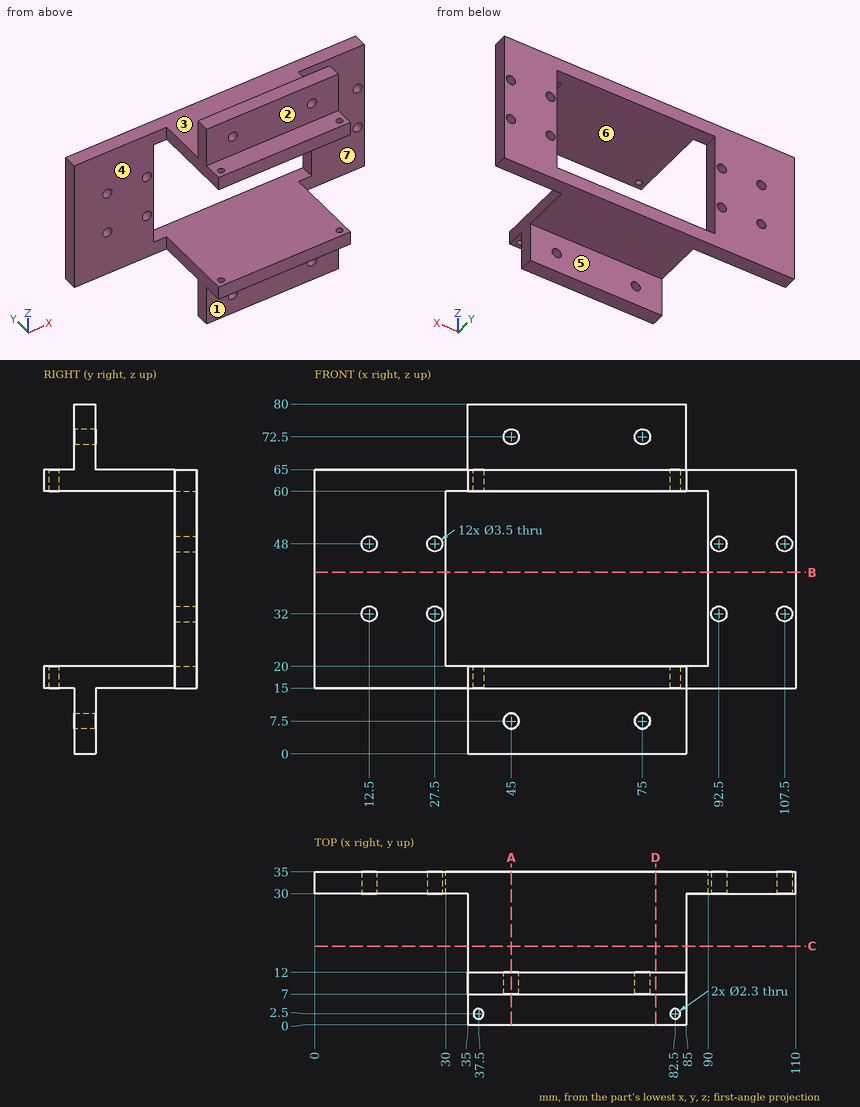
Could you check a few things on this drawing? It's one solid part, dimensions in mm from its lowest x, y, z. A direction names the side the tool comes from. Coordinates: 2 decimals unless noted, no trailing zeros. Order: outer loops, then holes, each group sorted by start corner. A loop starts at its lowest first (then second) coordinate and runs counter-clockwise, first axis right, second up. Notation, with made-up numbers: (30, -27) - (72, -27) arc R12 cw to (72, -9) - close; hole circle Ø11 at (12.25, 60). An arc over 180 degrees is marked (long way). One line per question, with ' | ' between items. Start each with the question number.
1. I'm going to push flat-ended pins straight in: pin 1 Ø5.5 at (x, y) = (51.5, 2) entering from -Z; pin 2 Ø3 at (x, z) = (12.5, 48) entering from +Y; pin 3 Ø10.5 at (x, z) = (9.5, 30) entering from -Y; pin 4 Ø12 at (x, z) = (49, 8) entering from -Y. Where does each tip first touch, or does it pass through?
2. If we section it at D-D (x = 78): Write out the boundary of the cut face in (y, z).
3. If we section it at B-B (z = 41.5): Write out the boundary of the cut face in (x, y), and give its area (3 significant figures).
4. If we mould it in two halves opening along X, with no side actions, what happens to the marked faces 6 and 7? For each: released by +X, released by -X, zero draft, split by the parting line, or undercut.
5. Which directions (+Z, -Z, +X, -X, +Y, -Y) give clear straight access to the entire face, cutting with the end or side of a thin tool? Please do the marked faces 1, 2, 3, 4 and 5.
6. Please list where these lines run through material, in increasing order: line 1 along X through (y, z) = (10.75, 72.5); line 2 along Z through (x, y) = (75, 9); line 3 along X through (y, z) = (31.45, 48). Write a range as [from, to].
7. If we section it at A-A (x = 45): Write out the boundary of the cut face in (y, z), and give its area (3 significant figures).
8. If we section it at C-C (y = 18): Write out the boundary of the cut face in (x, z).
Model answer:
1) pin 1: stops at z = 15 | pin 2: passes through | pin 3: stops at y = 30 | pin 4: stops at y = 7
2) outline: (0, 15) - (7, 15) - (7, 0) - (12, 0) - (12, 15) - (35, 15) - (35, 20) - (0, 20) - close; (0, 60) - (35, 60) - (35, 65) - (12, 65) - (12, 80) - (7, 80) - (7, 65) - (0, 65) - close
3) outline: (0, 30) - (30, 30) - (30, 35) - (0, 35) - close; (90, 30) - (110, 30) - (110, 35) - (90, 35) - close | area: 250 mm²
4) face 6: undercut | face 7: zero draft
5) face 1: -Z, +X, -X, -Y | face 2: +Z, +X, -X, -Y | face 3: +Z, +X, -X, +Y | face 4: +Z, -Z, -X, -Y | face 5: -Z, +X, -X, +Y
6) line 1: x = [35, 43.25], [46.75, 73.25], [76.75, 85] | line 2: z = [0, 5.75], [9.25, 20], [60, 70.75], [74.25, 80] | line 3: x = [0, 10.75], [14.25, 25.75], [29.25, 30], [90, 90.75], [94.25, 105.75], [109.25, 110]
7) outline: (0, 15) - (7, 15) - (7, 9.25) - (12, 9.25) - (12, 15) - (35, 15) - (35, 20) - (0, 20) - close; (0, 60) - (35, 60) - (35, 65) - (12, 65) - (12, 70.75) - (7, 70.75) - (7, 65) - (0, 65) - close; (7, 0) - (12, 0) - (12, 5.75) - (7, 5.75) - close; (7, 74.25) - (12, 74.25) - (12, 80) - (7, 80) - close | area: 465 mm²
8) outline: (35, 15) - (85, 15) - (85, 20) - (35, 20) - close; (35, 60) - (85, 60) - (85, 65) - (35, 65) - close
